Solid Edge part; units mm, degrees
sketch "Sketch1" plane through (0, 0, 0) normal (0, -1, 0) x (1, 0, 0)
  line L0 (0, 0) -> (20, 0)
  line L1 (20, 0) -> (20, 37)
  line L2 (20, 37) -> (0, 37)
  line L3 (0, 37) -> (0, 0)
extrude "Protrusion1" add sketch "Sketch1" along normal blind 20
sketch "Sketch2" plane through (20, -10, 18.5) normal (1, 0, 0) x (0, 1, 0)
  line L0 (5, -13.5) -> (5, 20.0916)
  line L1 (5, -13.5) -> (-5, -13.5)
  line L2 (-5, -13.5) -> (-5, 24.1099)
extrude "Cutout1" cut sketch "Sketch2" against normal blind 44.45 material side at (20, -5.05, 21.7958)
sketch "Sketch3" plane through (10, -10, 0) normal (0, 0, -1) x (0, 1, 0)
  circle A0 centre (0, 0) radius 9
extrude "Protrusion2" add sketch "Sketch3" along normal blind 15
chamfer "Chamfer1" distance 0.5 angle 45 1 edges at (10, -19, -15)
hole "Hole1" at (10, -10, -15) direction (0, 0, 1) diameter 8.5 end through all
hole "Hole_2" at (10, -20, 25) direction (0, 1, 0) diameter 10 end through all
sketch "Sketch4" plane through (10, -10, 18.5) normal (1, 0, 0) x (0, 1, 0)
  line L0 (10.8209, 15.5) -> (5, 18.5)
  line L1 (-5, 18.5) -> (5, 18.5)
  line L2 (-10.8209, 15.5) -> (-5, 18.5)
revolve "RevolvedCutout1" cut sketch "Sketch4" angle 70 mid plane about axis through (10, -5, 5) along (0, -1, 0) material side at (10, -2.0666, 35.5444)
properties part number "45644"
Read the model definition and answer for the solid it produces. Units are mm, in the model's axes. A direction names the side the tool comes from. Round coordinates to 2 decimals unless told otherwise and drop trailing zeros. Order: outer loops, then holes, each group sorted by start corner. A loop starts at its lowest first (then second) coordinate and runs counter-clockwise, first axis right, second up.
1) The mould has two halves that part along X. Classify faces 4 (the face through (10, 0, 17)), 5 (the face through (5.85, -10.92, -5.14)), 6 (the face through (0, -3, 14)): released by +X, released by -X, zero draft, split by the parting line, or undercut.
2) Flat-ended cylindrical pins translate along their axes: pin 1 (5 mm diameter, centred on x = 11, y = -9, fed in from +Z); pin 2 (4 mm diameter, centred on y = -10.5, z = -8.5, fed in from +X); pin 3 (1.5 mm diameter, centred on x = 9.5, y = -6, fed in from +Z); pin 4 (5 mm diameter, centred on y = -4, z = -8.5, fed in from -X). Find the tip coordinate at first contact, or state that the pin passes through.
3) The part is cut by section C-C on x = 10. Write down the section's boundary in (y, z).
4) Straight lines are drawn through the part: L1, parallel to Y at x = 18.75, z = 21; L2, parallel to X at y = -16.4, z = 25; L3, parallel to X at y = -10.25, z = -10. For each, find the intervals that lie inside material, in ascending order.
5) The part is cut by section D-D on z = 18.5. Write down the section's boundary in (x, y), plus the area to 3 significant figures.
6) For faces 1 (the face through (10, -15, 17)), 2 (the face through (10.149, -2.535, 35.729)), 3 (the face through (18.786, -11.951, -7.148)), determine the directions among +Z, -Z, +X, -X, +Y, -Y from which every point of the face is accessible in a straight line to the end or side of a thin tool.
7) The part is cut by section A-A on z = 25. Write down the section's boundary in (x, y).
8) The part is cut by section B-B on y = -10. Write down the section's boundary in (x, z).
Resolved:
1. face 4: zero draft
1. face 5: undercut
1. face 6: released by -X
2. pin 1: passes through
2. pin 2: stops at x = 19
2. pin 3: stops at z = 5
2. pin 4: stops at x = 1.71
3. outline: (-20, 0) - (-19, 0) - (-19, -14.5) - (-18.5, -15) - (-14.25, -15) - (-14.25, 5) - (-15, 5) - (-15, 20) - (-20, 20) - close; (-20, 30) - (-15, 30) - (-15, 37) - (-20, 34.42) - close; (-5.75, -15) - (-1.5, -15) - (-1, -14.5) - (-1, 0) - (0, 0) - (0, 20) - (-5, 20) - (-5, 5) - (-5.75, 5) - close; (-5, 30) - (0, 30) - (0, 34.42) - (-5, 37) - close
4. L1: y = -20 to -15, -5 to 0
4. L2: x = 0 to 5, 15 to 20
4. L3: x = 1 to 5.76, 14.24 to 19
5. outline: (0, -20) - (20, -20) - (20, -15) - (0, -15) - close; (0, -5) - (20, -5) - (20, 0) - (0, 0) - close
5. area: 200 mm2
6. face 1: +Z, +X, -X
6. face 2: +Z, +Y
6. face 3: -Z
7. outline: (0, -20) - (5, -20) - (5, -15) - (0, -15) - close; (0, -5) - (5, -5) - (5, 0) - (0, 0) - close; (15, -20) - (20, -20) - (20, -15) - (15, -15) - close; (15, -5) - (20, -5) - (20, 0) - (15, 0) - close
8. outline: (0, 0) - (1, 0) - (1, -14.5) - (1.5, -15) - (5.75, -15) - (5.75, 5) - (0, 5) - close; (14.25, -15) - (18.5, -15) - (19, -14.5) - (19, 0) - (20, 0) - (20, 5) - (14.25, 5) - close
